Geometry check sheet. Reference: the model listing, model coordinates, mm. Face numbers are marked on the shaded views. A direction names the side the tool comes from. Give positions to 0.01 mm unless a question says otherwise; leave off trailing zeros. Write each loop counter-clockwise with the first axis right and the second up, starting at its lowest first coordinate (ties: lowest second). Pieces come first, ordered by that corner, then holes. Notation, with made-up numbers: M 37,-15.75 L 49,-15.75 A20 ccw 49,7.25 Z; hole C -35.75,54.25 d9. An arc over 180 degrees is marked long. One line per item, written item: value. Start each with the question number.
1. Cross-section at A-A on x = -7.78. Record the cut outline in (y, z).
2. Cross-section at B-B on y = -8.87. Record the cut outline in (x, z).
3. Tool access check on the marked faces 4, 5, 6 and 7. Record the directions out of +Z, -Z, +X, -X, +Y, -Y that give a thin tool (end or side, any length) a straight path to the whole face; none if there is none.
4. Scan lines: line 1 (Y direction, x = 21.41, z = 56.85); line 2 (X direction, y = 3.65, z = -4.5); line 3 (Y direction, x = -12.5, z = -3.5). Record each from-to range of solid material in increasing order.
5. Gauge pin test, flat ends, axial feed: pin 1 (8 mm diameter, centred on y = -1.5, z = 2, fed in from +X); pin 2 (2 mm diameter, centred on x = 8, z = 49, fed in from +Y); pin 3 (4 mm diameter, centred on x = -3, z = -7, fed in from +Y). Record the tip position at first contact, or that the pin passes through.
6. Cross-section at D-D on x = 13. Record the cut outline in (y, z).
7. Cross-section at C-C on y = -2.25. Record the cut outline in (x, z), then the cut area to 3 significant figures.
8. Release check for a two-part mould opening along X. For the marked faces 1, 2 and 3 record: pulls with the +X half, pulls with the -X half, needs draft (parallel to the pull), parting line crosses it, or undercut.
from build123d import *

# Parameters (mm, degrees)
SKETCH_1_W          = 18
SKETCH_1_H          = 10
EXTRUDE_1_DEPTH     = 16.5
SKETCH_2_W          = 8
SKETCH_2_H          = 3.1
CUT_EXTRUDE_1_DEPTH = 40
SKETCH_3_R          = 1.65
CUT_EXTRUDE_2_DEPTH = 20
SKETCH_5_W          = 6
SKETCH_5_H          = 8
CUT_EXTRUDE_3_DEPTH = 20
SKETCH_6_W          = 30
SKETCH_6_H          = 5
EXTRUDE_2_DEPTH     = 47
SKETCH_7_W          = 46
SKETCH_7_H          = 22
SKETCH_7_R          = 0.91
EXTRUDE_3_DEPTH     = 2
SKETCH_8_W          = 18
SKETCH_8_H          = 7
CUT_EXTRUDE_4_DEPTH = 10


with BuildPart() as part:
    # 草图1 → 凸台-拉伸1 (new, symmetric)
    with BuildSketch(Plane(origin=(0, 0, 0), x_dir=(0, 0, -1), z_dir=(1, 0, 0))):
        Rectangle(SKETCH_1_W, SKETCH_1_H)
    extrude(amount=EXTRUDE_1_DEPTH, both=True)

    # 草图2 → 切除-拉伸1 (cut)
    with BuildSketch(Plane.ZY.offset(16.5)):
        with Locations((-5, 0)):
            Rectangle(SKETCH_2_W, SKETCH_2_H)
    extrude(amount=-CUT_EXTRUDE_1_DEPTH, mode=Mode.SUBTRACT)

    # 草图3 → 切除-拉伸2 (cut)
    with BuildSketch(Plane(origin=(0, 5, 0), x_dir=(1, 0, 0), z_dir=(0, 1, 0))):
        with Locations(Location((-7.78, 4.5, 0), (0, 0, 270))):
            Circle(SKETCH_3_R)
        with Locations(Location((7.78, 4.5, 0), (0, 0, 270))):
            Circle(SKETCH_3_R)
    extrude(amount=-CUT_EXTRUDE_2_DEPTH, mode=Mode.SUBTRACT)

    # 草图5 → 切除-拉伸3 (cut)
    with BuildSketch(Plane(origin=(0, 5, 0), x_dir=(1, 0, 0), z_dir=(0, 1, 0))):
        with Locations((0, 9)):
            Rectangle(SKETCH_5_W, SKETCH_5_H)
    extrude(amount=-CUT_EXTRUDE_3_DEPTH, mode=Mode.SUBTRACT)

    # 草图6 → 凸台-拉伸2 (add)
    with BuildSketch(Plane.XY.offset(9)):
        with Locations((0, -2.5)):
            Rectangle(SKETCH_6_W, SKETCH_6_H)
    extrude(amount=EXTRUDE_2_DEPTH)

    # 草图7 → 凸台-拉伸3 (add)
    with BuildSketch(Plane.XY.offset(56)):
        Rectangle(SKETCH_7_W, SKETCH_7_H)
        with Locations((-21.41, 8.87)):
            Circle(SKETCH_7_R, mode=Mode.SUBTRACT)
        with Locations(Location((21.41, 8.87, 0), (0, 0, 180))):
            Circle(SKETCH_7_R, mode=Mode.SUBTRACT)
        with Locations((21.41, -8.87)):
            Circle(SKETCH_7_R, mode=Mode.SUBTRACT)
        with Locations(Location((-21.41, -8.87, 0), (0, 0, 180))):
            Circle(SKETCH_7_R, mode=Mode.SUBTRACT)
    extrude(amount=EXTRUDE_3_DEPTH)

    # 草图8 → 切除-拉伸4 (cut)
    with BuildSketch(Plane.XY.offset(58)):
        with Locations((0, 7.5)):
            Rectangle(SKETCH_8_W, SKETCH_8_H)
        with Locations((0, -7.5)):
            Rectangle(SKETCH_8_W, SKETCH_8_H)
    extrude(amount=-CUT_EXTRUDE_4_DEPTH, mode=Mode.SUBTRACT)


solid = part.part
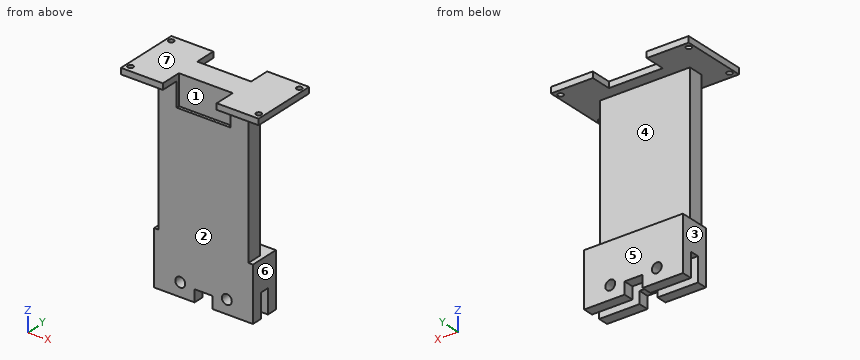
Report:
1. outline: M -5,-9 L -1.55,-9 L -1.55,-6.15 L -5,-6.15 Z; M -5,-2.85 L -1.55,-2.85 L -1.55,-1 L 1.55,-1 L 1.55,-2.85 L 5,-2.85 L 5,9 L 0,9 L 0,56 L 4,56 L 4,58 L -4,58 L -4,48 L -5,48 Z; M 1.55,-9 L 5,-9 L 5,-6.15 L 1.55,-6.15 Z
2. outline: M -23,56 L -22.32,56 L -22.32,58 L -23,58 Z; M -20.5,56 L -9,56 L -9,58 L -20.5,58 Z; M 9,56 L 20.5,56 L 20.5,58 L 9,58 Z; M 22.32,56 L 23,56 L 23,58 L 22.32,58 Z
3. face 4: +X, -X, +Y
3. face 5: -Z, +X, -X, +Y
3. face 6: -Z, +X, +Y, -Y
3. face 7: +Z, +X, -X, +Y, -Y
4. line 1: y = -11 to -9.78, -7.96 to 7.96, 9.78 to 11
4. line 2: x = -16.5 to -9.43, -6.13 to 6.13, 9.43 to 16.5
4. line 3: y = -5 to -1.55, 1.55 to 5
5. pin 1: stops at x = 16.5
5. pin 2: stops at y = 0
5. pin 3: stops at y = 5
6. outline: M -11,56 L -5,56 L -5,-9 L -1.55,-9 L -1.55,-1 L 1.55,-1 L 1.55,-9 L 5,-9 L 5,9 L 0,9 L 0,56 L 11,56 L 11,58 L -11,58 Z
7. outline: M -23,56 L -15,56 L -15,9 L -16.5,9 L -16.5,-9 L -3,-9 L -3,-5 L 3,-5 L 3,-9 L 16.5,-9 L 16.5,9 L 15,9 L 15,56 L 23,56 L 23,58 L -23,58 Z; hole C -7.78,-4.5 d3.3; hole C 7.78,-4.5 d3.3
7. area: 2,050 mm^2
8. face 1: undercut
8. face 2: needs draft
8. face 3: pulls with the -X half
